For this review, take the finished solid that the model builds, in its own axes (mm). Face numbers are marked on the shaded views. A direction names the side the tool comes from. Round coordinates to 2 decimals unless told otherwise and drop trailing zeros. Order: outer loops, then holes, each group sorted by start corner. A loop starts at its lowest first (then second) coordinate and runs counter-clockwise, first axis right, second up. Notation, with made-up numbers: M -13.5,-8 L -0.5,-8 A21 cw -0.5,17 Z; hole C 8.25,69.5 d10. An arc over 180 degrees is marked long. Answer as a JSON object with one key per item and string values.
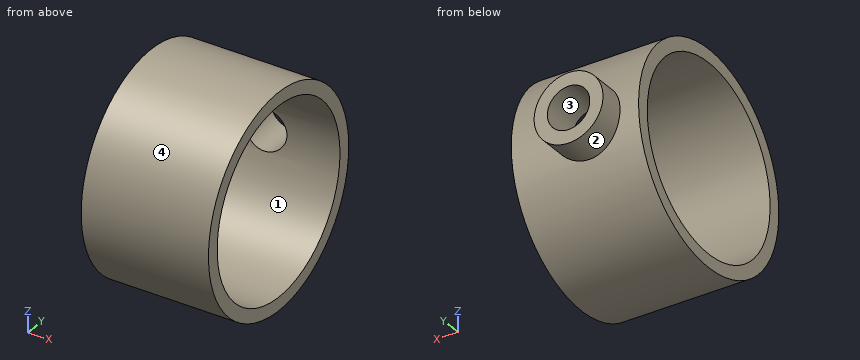
from build123d import *

# Parameters (mm, degrees)
SKETCH_10_R         = 1.3
EXTRUDE_1_DEPTH     = 1.3
SKETCH_11_R         = 0.8
CUT_EXTRUDE_2_DEPTH = 5.65


with BuildPart() as part:
    # 草图1 → 旋转1 (revolve)
    with BuildSketch(Plane.XY):
        Polygon((3.380941288, 3.525), (4.357609697, 3.525), (4.769072518, 3.525), (8.180941288, 3.525), (8.180941288, 4.025), (7.380941288, 4.025), (3.380941288, 4.025), align=None)
    revolve(axis=Axis((0, 0, 0), (1, 0, 0)))

    # 草图10 → 凸台-拉伸1 (add)
    with BuildSketch(Plane(origin=(0, 5, 0), x_dir=(1, 0, 0), z_dir=(0, 1, 0))):
        with Locations((5.380941288, 0)):
            Circle(SKETCH_10_R)
    extrude(amount=-EXTRUDE_1_DEPTH)

    # 草图11 → 切除-拉伸2 (cut, symmetric)
    with BuildSketch(Plane(origin=(0, 5, 0), x_dir=(1, 0, 0), z_dir=(0, 1, 0))):
        with Locations((5.380941288, 0)):
            Circle(SKETCH_11_R)
    extrude(amount=CUT_EXTRUDE_2_DEPTH, both=True, mode=Mode.SUBTRACT)


solid = part.part
1) Add section A-A on y = 0. State the section outline as (x, z) points (3 decimals).
Geometry check:
{"outline": "M 3.381,-4.025 L 8.181,-4.025 L 8.181,-3.525 L 3.381,-3.525 Z; M 3.381,3.525 L 8.181,3.525 L 8.181,4.025 L 3.381,4.025 Z"}
2) Add section C-C on z = -3. State the section outline as (x, y) points.
Geometry check:
{"outline": "M 3.38,-2.68 L 8.18,-2.68 L 8.18,-1.85 L 3.38,-1.85 Z; M 3.38,1.85 L 8.18,1.85 L 8.18,2.68 L 3.38,2.68 Z"}
3) Mouldability with a two-part tool opening along Z and no side actions: class the marked faces 3 and 4 as +Z half, -Z half, draft (parallel to the pull), parting line (faces both ways), or undercut.
Geometry check:
{"face 3": "undercut", "face 4": "parting line"}
4) Insertion check: P1, Ø1.4, axis at x = 5.38, z = 0, coming from the +Y side; P2, Ø1.5, axis at x = 6.5, y = -1, coming from the +Z side. Each pin has a flat end and moves straight along its axis. Give the tip position at first contact, or say it passes through.
Geometry check:
{"P1": "stops at y = -3.45", "P2": "stops at z = 4.02"}
5) Add section D-D on x = 7.85. State the section outline as (y, z) points (3 decimals), and give its area (3 significant figures).
Geometry check:
{"outline": "C 0,0 d8.05; hole C 0,0 d7.05", "area": "11.9 mm²"}
6) Add section B-B on z = 0. State the section outline as (x, y) points (3 decimals), and give its area (4 significant figures).
Geometry check:
{"outline": "M 3.381,-4.025 L 8.181,-4.025 L 8.181,-3.525 L 3.381,-3.525 Z; M 3.381,3.525 L 4.581,3.525 L 4.581,5 L 4.081,5 L 4.081,4.025 L 3.381,4.025 Z; M 6.181,3.525 L 8.181,3.525 L 8.181,4.025 L 6.681,4.025 L 6.681,5 L 6.181,5 Z", "area": "4.975 mm²"}
7) Machinability: for the marked faces 1 and 2, which of the approach directions +Z, -Z, +X, -X, +Y, -Y give a long, thin tool a straight path to every point of the face, cutting with its end or side? Answer none if there is none.
Geometry check:
{"face 1": "+X, -X", "face 2": "+Y"}
8) For L1, parallel to Z at x = 4.55, y = 0 (3 decimals); L2, parallel to Z at x = 4, y = 0.75; L3, parallel to Y at x = 6.8, z = 1.75, list the stretches that pass through material, from the lowest coordinate up.
Geometry check:
{"L1": "z = -4.025 to -3.525, 3.525 to 4.025", "L2": "z = -3.95 to -3.44, 3.44 to 3.95", "L3": "y = -3.62 to -3.06, 3.06 to 3.62"}
